The figure shows three views and two pictorial views of one solid part (mm, origin at its lowest corner). Answer the questions. Round coordinates to 2 decimals unless told otherwise and drop trailing zeros. Order: outer loops, then holes, each group sorted by start corner. A loop starts at its lowest first (then second) coordinate and runs counter-clockwise, first axis right, second up. Notation, with made-up numbers: (10, 43.5) -> (39, 43.5) arc R31 ccw to (39, 78.5) -> close; hole circle Ø10 at (21.5, -6). An arc over 180 degrees is marked (long way). Return JSON: item names as keys, results as strings. Group by question number.
(1) Each of these flat-tipped pins is pushed along its axis until it touches: pin 1 (5 mm diameter, centred on x = 156, y = 74.5, fed in from -Z); pin 2 (2.5 mm diameter, centred on x = 161.5, z = 2, fed in from +Y). Where does it stop, or does it pass through?
(2) Consider line 1 (X direction, y = 180, z = 2.35); line 2 (X direction, y = 5, z = 3.55); line 3 (Y direction, x = 10, z = 1.85). Determine where each line is inside the solid, lowest interval first. Write a range as [from, to].
(3) The part is cut by section D-D (z = 0.9). Determine the outline of the cut face in (x, y), plus the area to 3 significant figures.
(4) The part is cut by section C-C (x = 10). Determine the outline of the cut face in (y, z), plus the area to 3 significant figures.
(5) The part is cut by section B-B (y = 5). Determine the outline of the cut face in (x, z), plus the area to 3 significant figures.
(6) The part is cut by section A-A (y = 180). Determine the outline of the cut face in (x, z), plus the area to 3 significant figures.
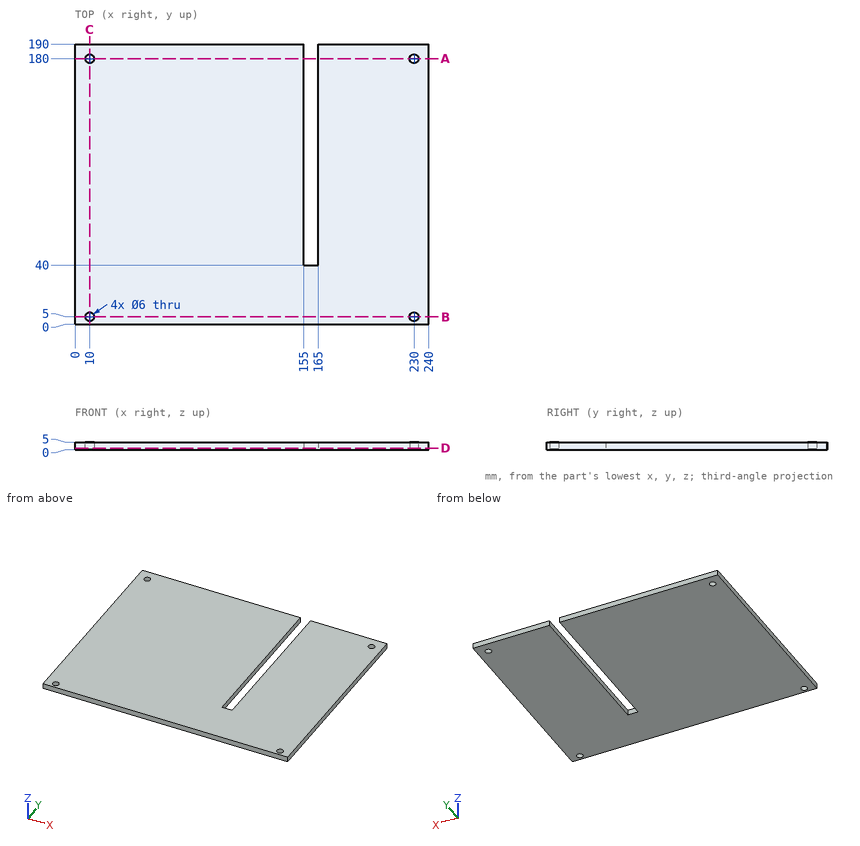
Answer below:
{
 "1": {"pin 1": "stops at z = 0", "pin 2": "stops at y = 40"},
 "2": {"line 1": "x = [0, 7], [13, 155], [165, 227], [233, 240]", "line 2": "x = [0, 7], [13, 227], [233, 240]", "line 3": "y = [0, 2], [8, 177], [183, 190]"},
 "3": {"outline": "(0, 0) -> (240, 0) -> (240, 190) -> (165, 190) -> (165, 40) -> (155, 40) -> (155, 190) -> (0, 190) -> close; hole circle Ø6 at (10, 5); hole circle Ø6 at (10, 180); hole circle Ø6 at (230, 5); hole circle Ø6 at (230, 180)", "area": "44,000 mm²"},
 "4": {"outline": "(0, 0) -> (2, 0) -> (2, 5) -> (0, 5) -> close; (8, 0) -> (177, 0) -> (177, 5) -> (8, 5) -> close; (183, 0) -> (190, 0) -> (190, 5) -> (183, 5) -> close", "area": "890 mm²"},
 "5": {"outline": "(0, 0) -> (7, 0) -> (7, 5) -> (0, 5) -> close; (13, 0) -> (227, 0) -> (227, 5) -> (13, 5) -> close; (233, 0) -> (240, 0) -> (240, 5) -> (233, 5) -> close", "area": "1,140 mm²"},
 "6": {"outline": "(0, 0) -> (7, 0) -> (7, 5) -> (0, 5) -> close; (13, 0) -> (155, 0) -> (155, 5) -> (13, 5) -> close; (165, 0) -> (227, 0) -> (227, 5) -> (165, 5) -> close; (233, 0) -> (240, 0) -> (240, 5) -> (233, 5) -> close", "area": "1,090 mm²"}
}
